```python
from build123d import *

# Parameters (mm, degrees)
BASE_EXTRUSION_DEPTH    = 3
ESQUISSE2_R             = 2
ENL_V_MAT_EXTRU_1_DEPTH = 3
CHANFREIN1_SIZE         = 0.5
ESQUISSE4_W             = 1
ESQUISSE4_H             = 0.5
BOSS_EXTRU_1_DEPTH      = 5


with BuildPart() as part:
    # Esquisse1 → Base-Extrusion (new body)
    with BuildSketch(Plane.XY):
        with BuildLine():
            Line((-10, 4), (10, 4))
            ThreePointArc((10, 4), (14, 0), (10, -4))
            Line((10, -4), (-10, -4))
            ThreePointArc((-10, -4), (-14, 0), (-10, 4))
        make_face()
    extrude(amount=BASE_EXTRUSION_DEPTH)

    # Esquisse2 → Enlèv. mat.-Extru.1 (cut)
    with BuildSketch(Plane.XY.offset(3)):
        with Locations(Location((0, 0, 0), (0, 0, 180))):
            Circle(ESQUISSE2_R)
    extrude(amount=-ENL_V_MAT_EXTRU_1_DEPTH, mode=Mode.SUBTRACT)

    # Chanfrein1
    chanfrein1_edges = [part.edges().sort_by_distance(p)[0] for p in [
        (0, -4, 0),
        (0, -4, 3),
        (14, 0, 0),
        (14, 0, 3),
        (-14, 0, 0),
        (-14, 0, 3),
        (0, 4, 0),
        (2, 0, 0),
        (0, 4, 3),
        (2, 0, 3),
    ]]
    chamfer(chanfrein1_edges, length=CHANFREIN1_SIZE)

    # Esquisse4 → Boss.-Extru.1 (add)
    with BuildSketch(Plane.XY):
        with Locations((0.5, 3.25)):
            Rectangle(ESQUISSE4_W, ESQUISSE4_H)
    extrude(amount=BOSS_EXTRU_1_DEPTH)


solid = part.part
```
Work out the finished part from the listing and answer in its coordinate system (mm). A direction names the side the tool comes from. Coordinates: 2 decimals unless noted, no trailing zeros. Loops run counter-clockwise (first coordinate to the right, second up) from the corner with the lowest first, then second, coordinate; pieces in that order, holes last. Notation, with made-up numbers: M 69,-34 L 80,-34 A17 ccw 80,-15 Z; hole C 50,-11 d10. An arc over 180 degrees is marked long. Use CSV: the item, a comma, the result in double quotes. Start each with the question number.
(1) Find section B-B, the plane x = -8.25. Give the vertices of the cut face in (y, z).
(2) Find section A-A, the plane z = 0.75. Give the vertices of the cut face in (x, y).
(3) Consider line 1 (Z direction, x = 9, y = 2.75); line 2 (Y direction, x = 0, z = 1.8); line 3 (X direction, y = -0.25, z = 1.4). Determine where each line is inside the solid, lowest interval first.
(4) Given pin 1 Ø2 at (x, y) = (2, 0.5) entering from +Z; pin 2 Ø0.5 at (x, z) = (0.5, 3.5) entering from +Y; pin 3 Ø1.5 at (x, z) = (3, 3.5) entering from -Y, each flat-ended and moving along its own axis, determine where each tip first touches the part or whether it passes through.
(5) For a pull along X with two mould halves and no side action, classify faces 4 (the face through (3, 0, 0)), 5 (the face through (14, 0, 1)), 6 (the face through (0, 2, 2)) as +X half, -X half, draft (parallel to the pull), parting line (faces both ways), or undercut.
(6) For faces 1 (the face through (0.5, 3.5, 4)), 2 (the face through (0.5, 3, 4)), 3 (the face through (-13.64, -0.08, 2.86)), determine the directions among +Z, -Z, +X, -X, +Y, -Y from which every point of the face is accessible in a straight line to the end or side of a thin tool.
Recorded:
1,outline,"M -4,0.5 L -3.5,0 L 3.5,0 L 4,0.5 L 4,2.5 L 3.5,3 L -3.5,3 L -4,2.5 Z"
2,outline,"M -10,-4 L 10,-4 A4 ccw 10,4 L -10,4 A4 ccw Z; hole C 0,0 d4"
3,line 1,"z = 0 to 3"
3,line 2,"y = -4 to -2, 2 to 4"
3,line 3,"x = -13.99 to -1.98, 1.98 to 13.99"
4,pin 1,"stops at z = 3"
4,pin 2,"stops at y = 3.5"
4,pin 3,"stops at y = -3.75"
5,face 4,"draft"
5,face 5,"+X half"
5,face 6,"undercut"
6,face 1,"+Z, +X, -X, +Y"
6,face 2,"+Z, +X, -X, -Y"
6,face 3,"+Z, -X"
